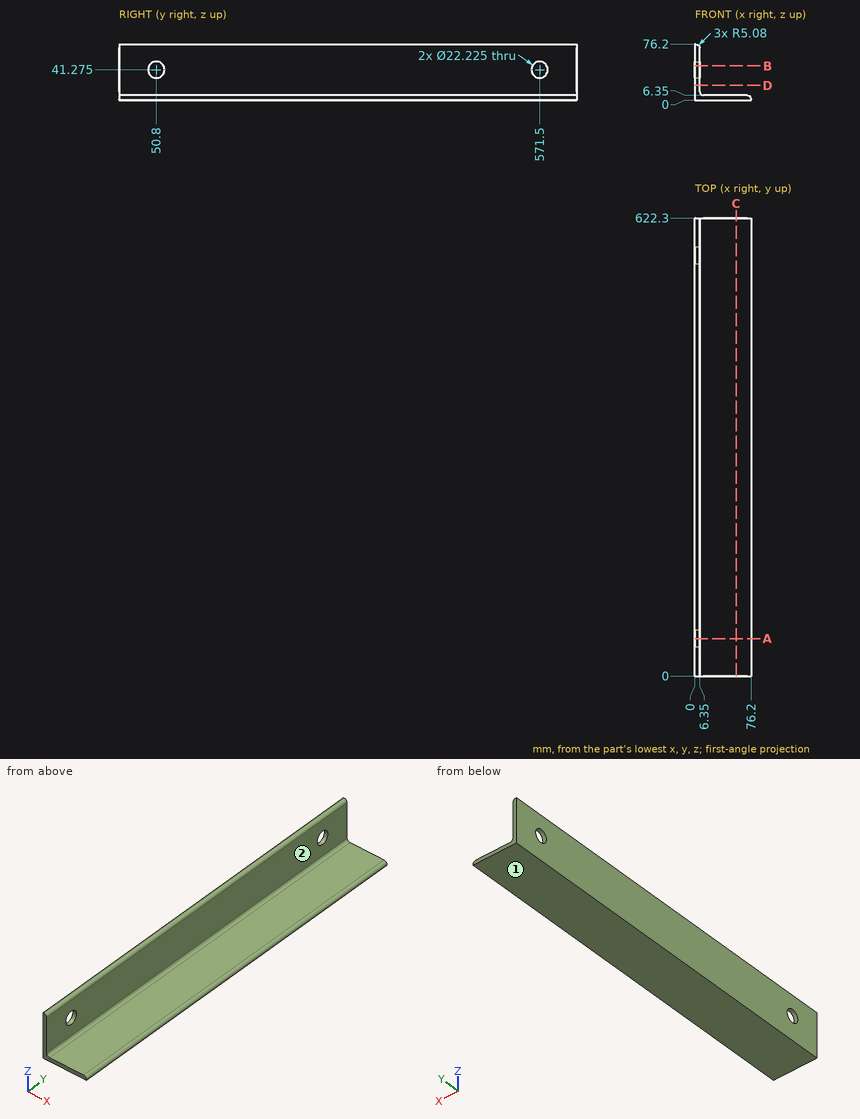
Geometry check sheet. Reference: drawing and pictorial views, mm from the part's lowest x, y, z. A direction names the side the tool comes from. Round coordinates to 2 decimals unless told otherwise and drop trailing zeros. Loops run counter-clockwise (first coordinate to the right, second up) from the corner with the lowest first, then second, coordinate; pieces in that order, holes last. Notation, with made-up numbers: (40, 88) - (54, 88) arc R28 cw to (54, 107) - close; hole circle Ø6 at (77.5, 42.25). An arc over 180 degrees is marked (long way). Use a Markdown table: item, result. Add a question column.
1. Section check D-D, the plane z = 20. Record the boundary of the cut face in (x, y).
2. Thickness scan on probe 1 along Z at (x, y) = (1.75, 50.8); probe 2 along Z at (x, y) = (2, 50.8); probe 3 along X at (y, z) = (462, 27.5). Record the ranges inside material, lowest first. Write a range as [from, to].
3. Section check A-A, the plane y = 50.8. Record the boundary of the cut face in (x, z).
4. Section check C-C, the plane x = 56. Record the boundary of the cut face in (y, z).
5. Access from +Z, -Z, +X, -X, +Y, -Y to the whole of each face (thin tool, end or side, straight path). Record for the marked faces 1 and 2.
6. Section check B-B, the plane z = 46.5. Record the boundary of the cut face in (x, y), plus the area to 3 significant figures.
7. Gauge pin test, flat ends, axial feed: pin 1 (1.5 mm diameter, centred on x = 20.5, y = 460.5, fed in from +Z); pin 2 (4 mm diameter, centred on y = 333.5, z = 49.5, fed in from +X). Record the tip position at first contact, or that the pin passes through.
Checks:
| question | item | result |
|---|---|---|
| 1 | outline | (0, 0) - (6.35, 0) - (6.35, 622.3) - (0, 622.3) - close |
| 2 | probe 1 | z = [0, 30.16], [52.39, 76.18] |
| 2 | probe 2 | z = [0, 30.16], [52.39, 76.15] |
| 2 | probe 3 | x = [0, 6.35] |
| 3 | outline | (0, 0) - (76.2, 0) - (76.2, 1.27) arc R5.08 ccw to (71.12, 6.35) - (11.43, 6.35) arc R5.08 cw to (6.35, 11.43) - (6.35, 30.16) - (0, 30.16) - close; (0, 52.39) - (6.35, 52.39) - (6.35, 71.12) arc R5.08 ccw to (1.27, 76.2) - (0, 76.2) - close |
| 4 | outline | (0, 0) - (622.3, 0) - (622.3, 6.35) - (0, 6.35) - close |
| 5 | face 1 | -Z, +X, -X, +Y, -Y |
| 5 | face 2 | +Z, +X, +Y, -Y |
| 6 | outline | (0, 0) - (6.35, 0) - (6.35, 40.99) - (0, 40.99) - close; (0, 60.61) - (6.35, 60.61) - (6.35, 561.69) - (0, 561.69) - close; (0, 581.31) - (6.35, 581.31) - (6.35, 622.3) - (0, 622.3) - close |
| 6 | area | 3,700 mm^2 |
| 7 | pin 1 | stops at z = 6.35 |
| 7 | pin 2 | stops at x = 6.35 |
